CAD build for the part. Positions are in the model's coordinates, mm. Face numbers are marked on the shaded views. A direction names the side the tool comes from. Round coordinates to 2 decimals unless told otherwise and drop trailing zeros. Write each loop counter-clockwise with the first axis right and the second up, starting at its lowest first coordinate (ties: lowest second). Pieces come first, ordered by that corner, then holes. Notation, with made-up numbers: (-10.75, 56) - (35.25, 56) arc R6 cw to (35.25, 62) - close; hole circle Ø3 at (41.25, -35). An arc over 180 degrees is marked (long way). Put each result on its own line as item: value. Start each with the question number.
Item 1: Pin check, flat tips, straight feed: pin 1 Ø1.8 at (x, y) = (-9, 2.5) entering from +Z; pin 2 Ø6.5 at (x, y) = (-8, -3) entering from +Z. Stop position of each tip, or through.
Item 2: Cut at B-B (y = -1.3). Give the cut face in (x, z).
Item 3: Drill centre lines: line 1 (Z direction, x = 2, y = -0.5); line 2 (X direction, y = 3.75, z = 17); line 3 (Z direction, x = 7, y = 0.75). Where is each one in solid material? Low to high. Write a range as from..to.
Item 4: Cut at C-C (x = 5.75). Give the cut face in (y, z).
Item 5: Cut at A-A (z = 5.2). Give the cut face in (x, y).
Item 6: 3-axis set-ups, long thin cutter, end or side, ignore diameter. For the marked faces 1, 2 and 3: which of +Z, -Z, +X, -X, +Y, -Y reach the whole face in a straight line?
Item 7: Cut at D-D (z = 15.5). Give the cut face in (x, y).
Solid Edge part; units mm, degrees
sketch "Sketch1" plane through (0, 0, 0) normal (0, 0, 1) x (1, 0, 0)
  line L0 (-11.2, -6) -> (11.2, -6)
  line L1 (11.2, -6) -> (11.2, 6)
  line L2 (11.2, 6) -> (-11.2, 6)
  line L3 (-11.2, 6) -> (-11.2, -6)
  dimension "D1" = 11.2
  dimension "D2" = 11.2
extrude "Protrusion1" add sketch "Sketch1" along normal blind 22.8
sketch "Sketch2" plane through (0, 0, 22.8) normal (0, 0, 1) x (1, 0, 0)
  arc A0 (-0.0038, 3) -> (-0.0038, -3) centre (-5.2, 0) ccw
  line L0 (-0.0038, -3) -> (0.55, -3)
  arc A1 (0.55, 3) -> (0.55, -3) centre (0.55, 0) cw
  line L1 (-0.0038, 3) -> (0.55, 3)
  dimension "D1" = 0.0038
extrude "Extrusionsausprägung_2" add sketch "Sketch2" along normal blind 4.5
sketch "Sketch3" plane through (-4.025, 0, 27.3) normal (0, 0, 1) x (1, 0, 0)
  circle A0 centre (-1.175, 0) radius 2.5
extrude "Extrusionsausprägung_3" add sketch "Sketch3" along normal blind 3
sketch "Sketch4" plane through (-11.2, 0, 11.2) normal (-1, 0, 0) x (0, -1, 0)
  circle A0 centre (0, -6) radius 0.6
  circle A1 centre (1.3, -6) radius 0.6
  circle A2 centre (-1.3, -6) radius 0.6
extrude "Extrusionsausprägung_4" add sketch "Sketch4" along normal blind 3
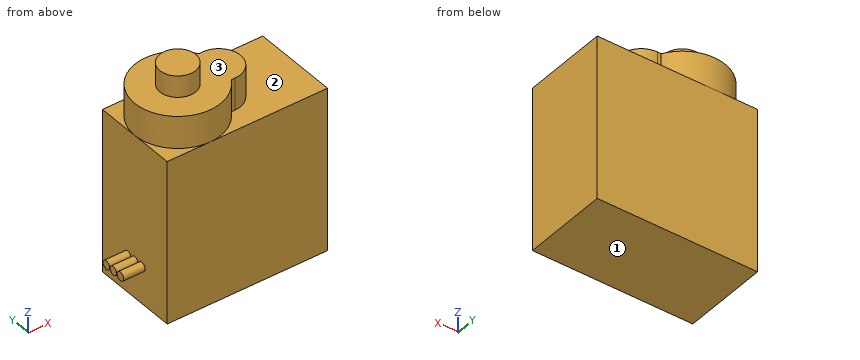
Output values:
1. pin 1: z = 27.3
1. pin 2: z = 30.3
2. outline: (-14.2, 4.6) - (-11.2, 4.6) - (-11.2, 0) - (11.2, 0) - (11.2, 22.8) - (3.25, 22.8) - (3.25, 27.3) - (-3.06, 27.3) - (-3.06, 30.3) - (-7.34, 30.3) - (-7.34, 27.3) - (-11.06, 27.3) - (-11.06, 22.8) - (-11.2, 22.8) - (-11.2, 5.8) - (-14.2, 5.8) - close
3. line 1: 0..27.3
3. line 2: -11.2..11.2
3. line 3: 0..22.8
4. outline: (-6, 0) - (6, 0) - (6, 22.8) - (-6, 22.8) - close
5. outline: (-14.2, -1.9) - (-11.2, -1.9) - (-11.2, -6) - (11.2, -6) - (11.2, 6) - (-11.2, 6) - (-11.2, 1.9) - (-14.2, 1.9) - (-14.2, 0.7) - (-11.2, 0.7) - (-11.2, 0.6) - (-14.2, 0.6) - (-14.2, -0.6) - (-11.2, -0.6) - (-11.2, -0.7) - (-14.2, -0.7) - close
6. face 1: -Z, +X, -X, +Y, -Y
6. face 2: +Z, +X
6. face 3: +Z
7. outline: (-11.2, -6) - (11.2, -6) - (11.2, 6) - (-11.2, 6) - close
